from build123d import *

# Parameters (mm, degrees)
PAD_DEPTH = 260
FILLET_R  = 1.7


with BuildPart() as part:
    # Sketch001 (on Sketch) → Pad (new body)
    with BuildSketch(Plane.XZ):
        with BuildLine():
            Line((11.041263, -4.271639), (10.832885, -3.08987))
            add(Edge.make_bspline(
                [(-6, 14.1661), (8.666682, 9.19528), (10.832885, -3.08987)],
                knots=[0, 0, 0, 1, 1, 1], degree=2))
            Line((-6, 14.1661), (-6, -7.276474))
            Line((-6, -7.276474), (11.041263, -4.271639))
        make_face()
        with BuildLine():
            Line((0, -5), (0, 7))
            Line((0, 7), (0.984808, 7.173648))
            add(Edge.make_bspline(
                [(0.984808, 7.173648), (7.306391, 5.39233), (8.86327, -3.437166)],
                knots=[0, 0, 0, 1, 1, 1], degree=2))
            Line((8.86327, -3.437166), (0, -5))
        make_face(mode=Mode.SUBTRACT)
    extrude(amount=PAD_DEPTH)

    # Fillet
    fillet_edges = [part.edges().sort_by_distance(p)[0] for p in [
        (8.86327, -130, -3.437166),
        (0, -130, -5),
        (11.041263, -130, -4.271639),
    ]]
    fillet(fillet_edges, radius=FILLET_R)


solid = part.part
Input: part model. Units: mm. Frame: model coordinates. Coordinates: 2 decimals unless noted, no trailing zeros.
Q1. Material intervals for line 1 (X direction, y = -72, z = 4.5); line 2 (Z direction, x = 4.75, y = -86.5); line 3 (X direction, y = -121.5, z = -1), sorted ascending.
Q2. Draft query along Z for faces 1 (the face through (0, -128, 2)), 2 (the face through (-6, -128, 4)), 3 (the face through (4.6, -128.18, -4.19)), 4 (the face through (1.57, -128.18, -5.94)). Return one class per face: +Z half, -Z half, draft (parallel to the pull), parting line (faces both ways), or undercut.
Q3. Contact query for flat-ended pins moving along their axis: pin 1 (1 mm diameter, centred on x = 8, y = -140, fed in from +Z); pin 2 (2 mm diameter, centred on x = 7.5, y = -167.5, fed in from -Z); pin 3 (1.5 mm diameter, centred on x = 5.5, y = -226, fed in from +Z). Output: stop coordinate, or through.
Working result:
1. line 1: x = -6 to 0, 5.39 to 7.86
1. line 2: z = -5.38 to -4.16, 5.13 to 8.14
1. line 3: x = -6 to 0, 8.3 to 10.36
2. face 1: undercut
2. face 2: draft
2. face 3: undercut
2. face 4: -Z half
3. pin 1: stops at z = 5.03
3. pin 2: stops at z = -5.07
3. pin 3: stops at z = 8.14
